```python
from build123d import *

# Parameters (mm, degrees)
SKETCH1_R           = 7.5
BOSS_EXTRUDE1_DEPTH = 44
CHAMFER1_SIZE       = 1
CHAMFER2_SIZE       = 1


with BuildPart() as part:
    # Sketch1 → Boss-Extrude1 (new body)
    with BuildSketch(Plane.XY):
        Circle(SKETCH1_R)
    extrude(amount=BOSS_EXTRUDE1_DEPTH)

    # Chamfer1
    chamfer1_edges = [part.edges().sort_by_distance(p)[0] for p in [
        (-7.5, 0, 0),
    ]]
    chamfer(chamfer1_edges, length=CHAMFER1_SIZE)

    # Chamfer2
    chamfer2_edges = [part.edges().sort_by_distance(p)[0] for p in [
        (-7.5, 0, 44),
    ]]
    chamfer(chamfer2_edges, length=CHAMFER2_SIZE)


solid = part.part
```
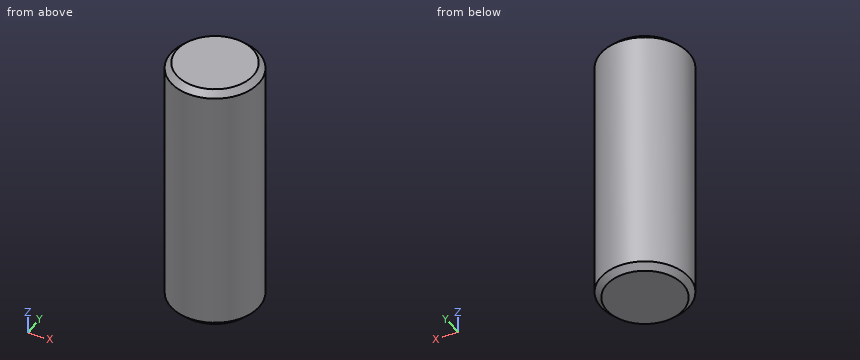
Geometry: final body of the model. Coordinates: model frame, mm. Coordinates: 2 decimals unless noted, no trailing zeros. Order: outer loops, then holes, each group sorted by start corner. A loop starts at its lowest first (then second) coordinate and runs counter-clockwise, first axis right, second up. Notation, with made-up numbers: (76, 75) -> (134, 75) arc R27 ccw to (134, 113) -> close; hole circle Ø6 at (89, 58.25). An arc over 180 degrees is marked (long way). Answer in a Markdown table with one row per item.
Item 1: Ray query, L1, parallel to X at y = 0.25, z = 2; L2, parallel to X at y = -2, z = 35; L3, parallel to Z at x = -5, y = -5.5. Return the intervals inside material, ascending.
Return value:
| item | result |
|---|---|
| L1 | x = -7.5 to 7.5 |
| L2 | x = -7.23 to 7.23 |
| L3 | z = 0.93 to 43.07 |
Item 2: Section A-A on z = 11.5. Output: boundary loops of the cut face in (x, y), plus the area to 3 significant figures.
Return value:
| item | result |
|---|---|
| outline | circle Ø15 at (0, 0) |
| area | 177 mm² |
Item 3: Contact query for flat-ended pins moving along their axis: P1, Ø4, axis at y = 5, z = 15, coming from the +X side; P2, Ø1.5, axis at x = 3.5, z = 16.5, coming from the -Y side; P3, Ø2, axis at y = 2, z = 38.5, coming from the -X side. Output: stop coordinate, or through.
Return value:
| item | result |
|---|---|
| P1 | stops at x = 6.87 |
| P2 | stops at y = -6.98 |
| P3 | stops at x = -7.43 |
